For this review, use the dimensioned drawing (mm, ordinates from the lowest corner) and the shaded views. A direction names the side the tool comes from. Coordinates: 2 decimals unless noted, no trailing zeros. Write each loop counter-clockwise with the first axis right and the second up, starting at its lowest first coordinate (ties: lowest second). Pieces come first, ordered by that corner, then holes.
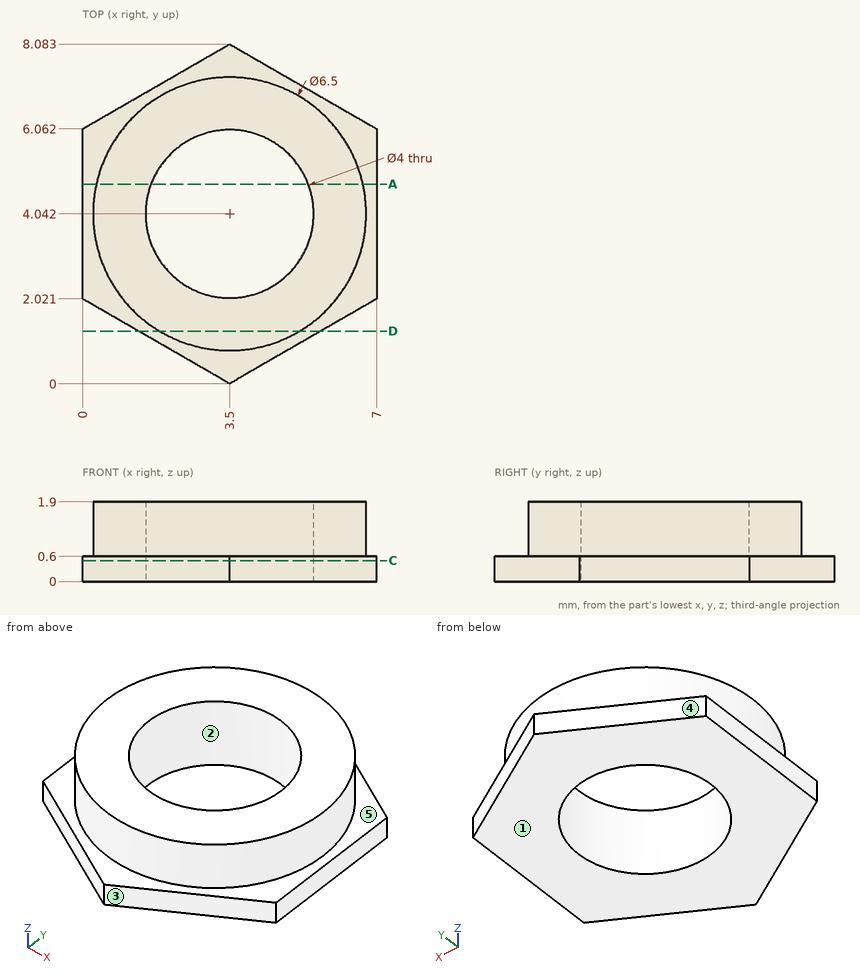
Item 1: Take a section at C-C, the plane z = 0.5. Write out the cut boundary in (x, y).
Solved:
outline: (0, 2.02) - (3.5, 0) - (7, 2.02) - (7, 6.06) - (3.5, 8.08) - (0, 6.06) - close; hole circle Ø4 at (3.5, 4.04)
Item 2: Take a section at D-D, the plane y = 1.25. Write out the cut boundary in (x, z) (1 decimal).
Solved:
outline: (1.3, 0) - (5.7, 0) - (5.7, 0.6) - (5.2, 0.6) - (5.2, 1.9) - (1.8, 1.9) - (1.8, 0.6) - (1.3, 0.6) - close
Item 3: To check wall thickness, follow line 1 along Y through (x, z) = (3.5, 1.5); line 2 along Z through (x, y) = (6.75, 5.5); line 3 along X through (y, z) = (4, 0.9). State the ranges of each line that lie inside material, in increasing order.
Solved:
line 1: y = 0.79 to 2.04, 6.04 to 7.29
line 2: z = 0 to 0.6
line 3: x = 0.25 to 1.5, 5.5 to 6.75
Item 4: Mouldability with a two-part tool opening along X and no side actions: class the marked faces 1, 2 and 3 as pulls with the +X half, pulls with the -X half, needs draft (parallel to the pull), parting line crosses it, or undercut.
Solved:
face 1: needs draft
face 2: undercut
face 3: pulls with the +X half
Item 5: For pin 1 (1.5 mm diameter, centred on x = 4.5, y = 4, fed in from +Z); pin 2 (1 mm diameter, centred on x = 1.5, z = 0.5, fed in from +Y), all flat-tipped, find the tip position at first contact; note any pin that passes through.
Solved:
pin 1: passes through
pin 2: stops at y = 7.22
Item 6: Take a section at A-A, the plane y = 4.75. Write out the cut boundary in (x, z).
Solved:
outline: (0, 0) - (1.63, 0) - (1.63, 1.9) - (0.33, 1.9) - (0.33, 0.6) - (0, 0.6) - close; (5.37, 0) - (7, 0) - (7, 0.6) - (6.67, 0.6) - (6.67, 1.9) - (5.37, 1.9) - close
Item 7: Machinability: for the marked faces 4 and 5, which of the approach directions +Z, -Z, +X, -X, +Y, -Y give a long, thin tool a straight path to every point of the face, cutting with its end or side? Answer none if there is none.
Solved:
face 4: +Z, -Z, -X, +Y
face 5: +Z
